Build history of the part. All positions in model axes, mm. A direction names the side the tool comes from. Give positions to 0.01 mm unless a question says otherwise; leave off trailing zeros. Order: outer loops, then holes, each group sorted by start corner. A loop starts at its lowest first (then second) coordinate and runs counter-clockwise, first axis right, second up. Notation, with made-up numbers: (30.25, 80) -> (46.25, 80) arc R25 cw to (46.25, 116) -> close; hole circle Ø11 at (59, -38.75). An arc over 180 degrees is marked (long way). One line per item, written item: value. Start each with the question number.
(1) Saw through at B-B on x = 0. Give the cut face in (y, z).
(2) Which spindle directions (+Z, -Z, +X, -X, +Y, -Y) get a long thin tool onto all of the face, cutting with end or side? Do faces 5 (the flat face through (1, 70, 38)), 6 (the flat face through (1, 50, 38)), 7 (the flat face through (-1, -70, 38)), 8 (the flat face through (-45, -60, 37)), 9 (the flat face through (45, 60, 38)). Say none if no direction does.
(3) Probe line 1 (Z direction, x = 0, y = -63.25); line 2 (Y direction, x = -17, z = 23.5); line 3 (Z direction, x = 74.5, y = -42.5). List the from-to ranges inside material, lowest first.
(4) Two-plate mould, pull along Z, no slides. Class faces 1 (the cylindrical face through (5.42, -59.86, 40.594)), 2 (the flat face through (-1, 1, 0)), 3 (the cylindrical face through (-13.44, 59.86, 43.92)), 4 (the flat face through (45, -60, 37)): +Z half, -Z half, draft (parallel to the pull), parting line (faces both ways), or undercut.
(5) Saw through at D-D on x = 31.5. Give the cut face in (y, z), plus the area to 3 significant figures.
(6) Saw through at C-C on z = 51.5. Give the cut face in (x, y).
(7) Pin check, flat tips, straight feed: pin 1 (4 mm diameter, centred on x = 28.5, y = 57, fed in from -Z); pin 2 (10 mm diameter, centred on y = 64, z = 30.5, fed in from +X); pin 3 (1 mm diameter, centred on x = -30.5, z = 54.5, fed in from +Y); pin 4 (1.5 mm diameter, centred on x = 44.5, z = 46.5, fed in from -Y). Stop position of each tip, or through.
(8) Saw through at A-A on z = 20.5. Give the cut face in (x, y), plus the area to 3 significant figures.
Autodesk Inventor part; units mm, degrees
ref_plane "Work Plane1" through (0, 50, 0) normal (0, 1, 0) x (-1, 0, 0)
ref_plane "YZ Plane" through (0, 0, 0) normal (1, 0, 0) x (0, 1, 0)
ref_plane "XY Plane" through (0, 0, 0) normal (0, 0, 1) x (1, 0, 0)
sketch "Sketch1" plane through (0, 0, 0) normal (0, 0, 1) x (1, 0, 0)
  circle A0 centre (0, 0) radius 90
  dimension "d0" = 180
extrude "Extrusion1" add sketch "Sketch1" along normal blind 10
ref_plane "Work Plane1" through (0, 50, 0) normal (0, 1, 0) x (-1, 0, 0)
sketch "Sketch2" plane through (0, 50, 0) normal (0, 1, 0) x (-1, 0, 0)
  line L0 (90, 10) -> (-90, 10)
  line L1 (0, 10) -> (0, 110) construction
  arc A0 (45, 65) -> (0, 110) centre (0, 65) ccw
  line L2 (45, 65) -> (45, 10)
  line L3 (45, 10) -> (0, 10)
  arc A1 (0, 110) -> (-45, 65) centre (0, 65) ccw
  line L4 (-45, 65) -> (-45, 10)
  line L5 (-45, 10) -> (0, 10)
  circle A2 centre (0, 65) radius 25
  point P0 (0, 0)
  dimension "d4" = 45
  dimension "d5" = 100
  dimension "d6" = 50
extrude "Extrusion2" add sketch "Sketch2" along normal blind 20
mirror "Mirror1" about plane through (0, 0, 0) normal (0, 1, 0) of "Extrusion2"
properties part number "Platform"
Results below:
1. outline: (-90, 0) -> (90, 0) -> (90, 10) -> (70, 10) -> (70, 40) -> (50, 40) -> (50, 10) -> (-50, 10) -> (-50, 40) -> (-70, 40) -> (-70, 10) -> (-90, 10) -> close; (-70, 90) -> (-50, 90) -> (-50, 110) -> (-70, 110) -> close; (50, 90) -> (70, 90) -> (70, 110) -> (50, 110) -> close
2. face 5: +Z, +X, -X, +Y
2. face 6: +Z, +X, -X
2. face 7: +Z, +X, -X, -Y
2. face 8: +Z, -X, +Y, -Y
2. face 9: +Z, +X, +Y, -Y
3. line 1: z = 0 to 40, 90 to 110
3. line 2: y = -70 to -50, 50 to 70
3. line 3: z = 0 to 10
4. face 1: undercut
4. face 2: -Z half
4. face 3: undercut
4. face 4: draft
5. outline: (-84.31, 0) -> (84.31, 0) -> (84.31, 10) -> (70, 10) -> (70, 97.14) -> (50, 97.14) -> (50, 10) -> (-50, 10) -> (-50, 97.14) -> (-70, 97.14) -> (-70, 10) -> (-84.31, 10) -> close
5. area: 5,170 mm²
6. outline: (-45, -70) -> (-21.04, -70) -> (-21.04, -50) -> (-45, -50) -> close; (-45, 50) -> (-21.04, 50) -> (-21.04, 70) -> (-45, 70) -> close; (21.04, -70) -> (45, -70) -> (45, -50) -> (21.04, -50) -> close; (21.04, 50) -> (45, 50) -> (45, 70) -> (21.04, 70) -> close
7. pin 1: stops at z = 0
7. pin 2: stops at x = 45
7. pin 3: stops at y = 70
7. pin 4: stops at y = -70
8. outline: (-45, -70) -> (45, -70) -> (45, -50) -> (-45, -50) -> close; (-45, 50) -> (45, 50) -> (45, 70) -> (-45, 70) -> close
8. area: 3,600 mm²
